from build123d import *

# Parameters (mm, degrees)
SKETCH_1_W          = 19
SKETCH_1_H          = 16
EXTRUDE_1_DEPTH     = 3.5
SKETCH_1_3_R        = 1.35
CUT_EXTRUDE_1_DEPTH = 19.145247312
CUT_EXTRUDE_START   = 1
SKETCH_1_4_R        = 2.4
SKETCH_1_4_R_2      = 1.35
CUT_EXTRUDE_2_DEPTH = 2.5
SKETCH_1_7_R        = 0.7
CUT_EXTRUDE_3_DEPTH = 19.145247312
SKETCH_1_18_R       = 0.95
CUT_EXTRUDE_8_DEPTH = 3
SKETCH_1_17_R       = 1.25
CUT_EXTRUDE_4_DEPTH = 19.145247312
SKETCH_2_W          = 9.8
SKETCH_2_H          = 4.5
CUT_EXTRUDE_5_DEPTH = 3
SKETCH_4_R          = 1.05
CUT_EXTRUDE_6_DEPTH = 2.8
SKETCH_5_R          = 2
EXTRUDE_2_DEPTH     = 3
CUT_EXTRUDE_START_2 = 3
SKETCH_5_3_R        = 0.3
CUT_EXTRUDE_7_DEPTH = 1.5


with BuildPart() as part:
    # 草图1 → 凸台-拉伸1 (new body)
    with BuildSketch(Plane(origin=(0, 0, 0), x_dir=(1, 0, 0), z_dir=(0, 1, 0))):
        with Locations((-4.5, 3)):
            Rectangle(SKETCH_1_W, SKETCH_1_H)
    extrude(amount=EXTRUDE_1_DEPTH)

    # 草图1<3> → 切除-拉伸1 (cut, through all)
    with BuildSketch(Plane(origin=(0, 0, 0), x_dir=(1, 0, 0), z_dir=(0, 1, 0))):
        with Locations(Location((0, 0, 0), (0, 0, 270))):
            Circle(SKETCH_1_3_R)
    extrude(amount=CUT_EXTRUDE_1_DEPTH, mode=Mode.SUBTRACT)

    # 草图1<4> → 切除-拉伸2 (cut)
    with BuildSketch(Plane(origin=(0, 0, 0), x_dir=(1, 0, 0), z_dir=(0, 1, 0)).offset(CUT_EXTRUDE_START)):
        with Locations(Location((0, 0, 0), (0, 0, 270))):
            Circle(SKETCH_1_4_R)
        with Locations(Location((0, 0, 0), (0, 0, 270))):
            Circle(SKETCH_1_4_R_2, mode=Mode.SUBTRACT)
    extrude(amount=CUT_EXTRUDE_2_DEPTH, mode=Mode.SUBTRACT)

    # 草图1<7> → 切除-拉伸3 (cut, through all)
    with BuildSketch(Plane(origin=(0, 0, 0), x_dir=(1, 0, 0), z_dir=(0, 1, 0))):
        with Locations(Location((4, 4, 0), (0, 0, 270))):
            Circle(SKETCH_1_7_R)
        with Locations(Location((-4, -4, 0), (0, 0, 270))):
            Circle(SKETCH_1_7_R)
        with Locations(Location((-4, 4, 0), (0, 0, 270))):
            Circle(SKETCH_1_7_R)
        with Locations(Location((4, -4, 0), (0, 0, 270))):
            Circle(SKETCH_1_7_R)
    extrude(amount=CUT_EXTRUDE_3_DEPTH, mode=Mode.SUBTRACT)

    # 草图1<18> → 切除-拉伸8 (cut)
    with BuildSketch(Plane(origin=(0, 0, 0), x_dir=(1, 0, 0), z_dir=(0, 1, 0))):
        with Locations(Location((4, 4, 0), (0, 0, 270))):
            Circle(SKETCH_1_18_R)
        with Locations(Location((-4, -4, 0), (0, 0, 270))):
            Circle(SKETCH_1_18_R)
        with Locations(Location((-4, 4, 0), (0, 0, 270))):
            Circle(SKETCH_1_18_R)
        with Locations(Location((4, -4, 0), (0, 0, 270))):
            Circle(SKETCH_1_18_R)
    extrude(amount=CUT_EXTRUDE_8_DEPTH, mode=Mode.SUBTRACT)

    # 草图1<17> → 切除-拉伸4 (cut, through all)
    with BuildSketch(Plane(origin=(0, 0, 0), x_dir=(1, 0, 0), z_dir=(0, 1, 0))):
        with Locations(Location((-3.9, 6.4, 0), (0, 0, 270))):
            Circle(SKETCH_1_17_R)
    extrude(amount=CUT_EXTRUDE_4_DEPTH, mode=Mode.SUBTRACT)

    # 草图2 → 切除-拉伸5 (cut)
    with BuildSketch(Plane(origin=(0, 3.5, 0), x_dir=(1, 0, 0), z_dir=(0, 1, 0))):
        with Locations((-0.3, 7.25)):
            Rectangle(SKETCH_2_W, SKETCH_2_H)
    extrude(amount=-CUT_EXTRUDE_5_DEPTH, mode=Mode.SUBTRACT)

    # 草图4 → 切除-拉伸6 (cut)
    with BuildSketch(Plane.XZ):
        with Locations(Location((-8.107149516, -2.554237014, 0), (0, 0, 270))):
            Circle(SKETCH_4_R)
    extrude(amount=-CUT_EXTRUDE_6_DEPTH, mode=Mode.SUBTRACT)

    # 草图5 → 凸台-拉伸2 (add)
    with BuildSketch(Plane.XZ):
        with Locations(Location((-12, 3, 0), (0, 0, 90))):
            Circle(SKETCH_5_R)
        with Locations(Location((-12, -9, 0), (0, 0, 270))):
            Circle(SKETCH_5_R)
        with Locations(Location((3, -9, 0), (0, 0, 270))):
            Circle(SKETCH_5_R)
    extrude(amount=EXTRUDE_2_DEPTH)

    # 草图5<3> → 切除-拉伸7 (cut)
    with BuildSketch(Plane.XZ.offset(CUT_EXTRUDE_START_2)):
        with Locations(Location((3, -9, 0), (0, 0, 270))):
            Circle(SKETCH_5_3_R)
        with Locations(Location((-12, -9, 0), (0, 0, 270))):
            Circle(SKETCH_5_3_R)
        with Locations(Location((-12, 3, 0), (0, 0, 270))):
            Circle(SKETCH_5_3_R)
    extrude(amount=-CUT_EXTRUDE_7_DEPTH, mode=Mode.SUBTRACT)


solid = part.part
Check sheet for the modelled part. Datum: model origin and axes. Units: mm. A direction names the side the tool comes from. Round coordinates to 2 decimals unless told otherwise and drop trailing zeros. Loops run counter-clockwise (first coordinate to the right, second up) from the corner with the lowest first, then second, coordinate; pieces in that order, holes last.
1. Set-up check for faces 4 (the cylindrical face through (3.574, 3.246, 3.445)), 5 (the flat face through (-8, 2.8, -3)), 6 (the cylindrical face through (2.024, 2.232, 1.29)), 7 (the flat face through (-13.6, 0, 4.5)): record each of +Z, -Z, +X, -X, +Y, -Y from which the full face is reachable in a straight line by a thin tool's end or side.
2. Gauge pin test, flat ends, axial feed: pin 1 Ø1.8 at (x, z) = (4, 4) entering from +Y; pin 2 Ø2.5 at (x, z) = (0.5, 0.5) entering from +Y; pin 3 Ø1 at (x, z) = (4.5, 4.5) entering from -Y. Record the tip position at first contact, or that the pin passes through.
3. Scan lines: probe 1 along X at (y, z) = (3.15, -4); probe 2 along Z at (x, y) = (-4, 3.1); probe 3 along Z at (x, y) = (-8, 0.5). Record each from-to range of solid material in increasing order.
4. Sectioned sample at A-A on x = 0. Record the boundary of the cut face in (y, z), and give its area (3 significant figures).
5. Sectioned sample at B-B on z = 0. Record the boundary of the cut face in (x, y), and give its area (3 significant figures).
6. Sectioned sample at C-C on y = 2. Record the boundary of the cut face in (x, z).
7. Sectioned sample at D-D on z = -6.4. Record the boundary of the cut face in (x, y).
8. Mould release check, pull along Z, two halves, no side actions. Record for faces 1 (the flat face through (4.5, 0, -10.6)), 2 (the flat face through (4.6, 2, -7)), 3 (the flat face through (-5, 2, -11)): released by +Z, released by -Z, zero draft, split by the parting line, or undercut.
Recorded:
1. face 4: +Y, -Y
1. face 5: -Y
1. face 6: +Y
1. face 7: +Z, -X, -Y
2. pin 1: stops at y = 3.5
2. pin 2: stops at y = 1
2. pin 3: stops at y = 0
3. probe 1: x = -14 to -4.7, -3.3 to 3.3, 4.7 to 5
3. probe 2: z = -11 to -9.5, -5 to -4.7, -3.3 to 3.3, 4.7 to 5
3. probe 3: z = -11 to -3.6, -1.51 to 5
4. outline: (0, -11) - (3.5, -11) - (3.5, -9.5) - (0.5, -9.5) - (0.5, -5) - (3.5, -5) - (3.5, -2.4) - (1, -2.4) - (1, -1.35) - (0, -1.35) - close; (0, 1.35) - (1, 1.35) - (1, 2.4) - (3.5, 2.4) - (3.5, 5) - (0, 5) - close
4. area: 27.8 mm2
5. outline: (-14, 0) - (-1.35, 0) - (-1.35, 1) - (-2.4, 1) - (-2.4, 3.5) - (-14, 3.5) - close; (1.35, 0) - (5, 0) - (5, 3.5) - (2.4, 3.5) - (2.4, 1) - (1.35, 1) - close
5. area: 51.8 mm2
6. outline: (-14, -11) - (5, -11) - (5, 5) - (-14, 5) - close; hole circle Ø2.1 at (-8.11, -2.55); hole (-5.2, -9.5) - (4.6, -9.5) - (4.6, -5) - (-5.2, -5) - close; hole circle Ø1.9 at (-4, -4); hole circle Ø1.9 at (-4, 4); hole circle Ø4.8 at (0, 0); hole circle Ø1.9 at (4, -4); hole circle Ø1.9 at (4, 4)
7. outline: (-14, 0) - (-5.15, 0) - (-5.15, 0.5) - (-5.2, 0.5) - (-5.2, 3.5) - (-14, 3.5) - close; (-2.65, 0) - (5, 0) - (5, 3.5) - (4.6, 3.5) - (4.6, 0.5) - (-2.65, 0.5) - close
8. face 1: zero draft
8. face 2: undercut
8. face 3: released by -Z
